Autodesk Inventor part; units mm, degrees
ref_plane "YZ Plane" through (0, 0, 0) normal (1, 0, 0) x (0, 1, 0)
ref_plane "XZ Plane" through (0, 0, 0) normal (0, 1, 0) x (-1, 0, 0)
ref_plane "XY Plane" through (0, 0, 0) normal (0, 0, 1) x (1, 0, 0)
sketch "スケッチ1" plane through (0, 0, 0) normal (0, 1, 0) x (-1, 0, 0)
  line L0 (-10, 8) -> (10, 8)
  line L1 (10, 8) -> (10, -8)
  line L2 (10, -8) -> (-10, -8)
  line L3 (-10, -8) -> (-10, 8)
  line L4 (-10, 8) -> (10, -8) construction
  line L5 (10, 8) -> (-10, -8) construction
  point P0 (0, 0)
  dimension "d0" = 20
  dimension "d1" = 16
extrude "プレート1" add sketch "スケッチ1" along normal blind 2
sketch "スケッチ2" plane through (12, 4, -8) normal (1, 0, 0) x (0, 1, 0)
  line L0 (0, 16) -> (0, 0)
  line L1 (0, 0) -> (16, 0)
  line L2 (16, 0) -> (16, 16)
  line L3 (16, 16) -> (0, 16)
edge flange "フランジ1" height 20 angle 90 thickness 2 bend radius 2 thickness toward (1, 0, 0) relief tear relief width 2 relief depth 1 edges at (10, 2, 0) wall of the first edge with corners at (12, 4, 8) (12, 4, -8) (12, 20, -8) (12, 20, 8)
bend "曲げ1"
corner "コーナー1"
sketch "スケッチ3" plane through (14, 20, 8) normal (1, 0, 0) x (0, 0, -1)
  line L0 (2.5, -4) -> (2.5, -13)
  arc A0 (2.5, -13) -> (5.5, -13) centre (4, -13) ccw
  line L1 (5.5, -13) -> (5.5, -4)
  arc A1 (5.5, -4) -> (2.5, -4) centre (4, -4) ccw
  line L2 (10.5, -4) -> (10.5, -13)
  arc A2 (10.5, -13) -> (13.5, -13) centre (12, -13) ccw
  line L3 (13.5, -13) -> (13.5, -4)
  arc A3 (13.5, -4) -> (10.5, -4) centre (12, -4) ccw
  line L4 (0, -16) -> (0, 0)
  line L5 (16, 0) -> (16, -16)
  line L6 (0, 0) -> (16, 0)
  line L7 (0, -16) -> (16, -16)
  point P0 (8, -20)
  dimension "d13" = 4
  dimension "d14" = 4
  dimension "d17" = 3
  dimension "d18" = 4
  dimension "d19" = 1.5
  dimension "d20" = 1.5
extrude "押し出し1" cut sketch "スケッチ3" against normal blind 10 contours A1 L1 A0 L0 | A3 L3 A2 L2
sketch "スケッチ4" plane through (0, 2, 0) normal (0, 1, 0) x (1, 0, 0)
  line L0 (-6, -1.5) -> (6, -1.5)
  arc A0 (6, -1.5) -> (6, 1.5) centre (6, 0) ccw
  line L1 (6, 1.5) -> (-6, 1.5)
  arc A1 (-6, 1.5) -> (-6, -1.5) centre (-6, 0) ccw
  line L2 (-10, -8) -> (-10, 8)
  line L3 (10, 8) -> (10, -8)
  point P0 (0, 0)
  dimension "d23" = 4
  dimension "d24" = 4
  dimension "d25" = 1.5
extrude "押し出し2" cut sketch "スケッチ4" against normal blind 10
equation "\"d2\" = Thickness"
equation "\"d3\" = BendReliefWidth"
equation "\"d4\" = BendReliefDepth"
equation "\"d5\" = MinimumRemnant"
equation "\"d6\" = TransitionRadius"
equation "\"d9\" = BendRadius"
equation "\"d10\" = CornerReliefSize"
equation "\"d11\" = GapSize"
equation "\"d12\" = JacobiRadiusSize"
equation "\"BendRadius\" = Thickness"
equation "\"BendReliefWidth\" = Thickness"
equation "\"BendReliefDepth\" = 0.5 * Thickness"
equation "\"CornerReliefSize\" = 4 * Thickness"
equation "\"MinimumRemnant\" = 2 * Thickness"
equation "\"TransitionRadius\" = BendRadius"
equation "\"JacobiRadiusSize\" = BendRadius"
equation "\"GapSize\" = Thickness"
properties part number "keyL_medium" material "アルミニウム 6061"
Could you check a few things on this model? Use its own coordinates, in mm. A direction names the side the tool comes from. Give positions to 0.01 mm unless a question says otherwise; leave off trailing zeros. Loops run counter-clockwise (first coordinate to the right, second up) from the corner with the lowest first, then second, coordinate; pieces in that order, holes last. Notation, with made-up numbers: M -21,21.5 L 20,21.5 A18 ccw 20,52.5 Z; hole C 58.25,3 d8. An arc over 180 degrees is marked long. Answer as a JSON object with one key per item and string values.
Q1. Suppose I cut it at D-D, the plane z = -6. List the corners of the cut face in (x, y) for me, plus the area to 3 significant figures.
Values found:
{"outline": "M -10,0 L 10,0 A4 ccw 14,4 L 14,20 L 12,20 L 12,4 A2 cw 10,2 L -10,2 Z", "area": "81.4 mm²"}
Q2. Suppose I cut it at B-B, the plane y = 10. List the corners of the cut face in (x, z) for me, plus the area to 3 significant figures.
Values found:
{"outline": "M 12,-8 L 14,-8 L 14,-5.5 L 12,-5.5 Z; M 12,-2.5 L 14,-2.5 L 14,2.5 L 12,2.5 Z; M 12,5.5 L 14,5.5 L 14,8 L 12,8 Z", "area": "20.0 mm²"}
Q3. If we mould it in two halves opening along Y, with no side actions, what happens to faces 5 (the flat face through (13, 11, 2.5)), 6 (the flat face through (0, 0, 2)), 7 (the flat face through (5.6, 1.8, 8))? For each: pulls with the +Y half, pulls with the -Y half, needs draft (parallel to the pull), parting line crosses it, or undercut.
Values found:
{"face 5": "undercut", "face 6": "pulls with the -Y half", "face 7": "needs draft"}
Q4. For P1, Ø5, axis at x = 3.5, z = -2, coming from the +Y side; P2, Ø6, axis at x = 8, z = -6, coming from the +Y side, each with a flat end and sliding along its axis, tell me the tip position at first contact or that it passes through.
Values found:
{"P1": "stops at y = 2", "P2": "stops at y = 2.27"}
Q5. Suppose I cut it at A-A, the plane z = -4. List the corners of the cut face in (x, y) for me.
Values found:
{"outline": "M -10,0 L 10,0 A4 ccw 14,4 L 14,5.5 L 12,5.5 L 12,4 A2 cw 10,2 L -10,2 Z; M 12,17.5 L 14,17.5 L 14,20 L 12,20 Z"}
Q6. If I drill on probe 1 along Z at (x, y) = (12.5, 16); probe 2 along X at (y, z) = (14.5, 0.75); probe 3 along Y at (x, z) = (5.25, 5.5), over which ranges is the centre line in solid material (lowest first)? Write a range as [from, to].
Values found:
{"probe 1": "z = [-8, -5.5], [-2.5, 2.5], [5.5, 8]", "probe 2": "x = [12, 14]", "probe 3": "y = [0, 2]"}
Q7. For faces 1 (the cylindrical face through (7.5, 1, 0)), 2 (the flat face through (12, 12, 0)), 3 (the flat face through (14, 12, 0)), 4 (the cylindrical face through (13, 5.5, 4)), which set-ups out of +Z, -Z, +X, -X, +Y, -Y let a thin tool reach every point of the face, with its end or its side?
Values found:
{"face 1": "+Y, -Y", "face 2": "+Z, -Z, -X, +Y", "face 3": "+Z, -Z, +X, +Y, -Y", "face 4": "+X, -X"}
Q8. Suppose I cut it at C-C, the plane x = 4.75. List the corners of the cut face in (y, z) for me.
Values found:
{"outline": "M 0,-8 L 2,-8 L 2,-1.5 L 0,-1.5 Z; M 0,1.5 L 2,1.5 L 2,8 L 0,8 Z"}
